```python
from build123d import *

# Parameters (mm, degrees)
SKETCH3_W           = 110
SKETCH3_H           = 180
BOSS_EXTRUDE1_DEPTH = 3
CUT_EXTRUDE1_REACH  = 107.518
SKETCH4_W           = 35
SKETCH4_H           = 55
CUT_EXTRUDE2_REACH  = 107.518
SKETCH5_R           = 1.5
FILLET1_R           = 10
FILLET2_R           = 10
SKETCH9_W           = 35
SKETCH9_H           = 3
BOSS_EXTRUDE2_DEPTH = 18.556788
BOSS_EXTRUDE3_START = -16.676438017
BOSS_EXTRUDE3_DEPTH = 35
CUT_EXTRUDE3_REACH  = 124.809
SKETCH16_W          = 10
SKETCH16_H          = 40
CHAMFER1_SIZE       = 10


# Read off the part's stored shape, not the designer's step: Boss-Extrude3
with BuildPart() as part:
    # Sketch3 → Boss-Extrude1 (new body)
    with BuildSketch(Plane(origin=(0, 0, 0), x_dir=(1, 0, 0), z_dir=(0, 1, 0))):
        Rectangle(SKETCH3_W, SKETCH3_H)
    extrude(amount=BOSS_EXTRUDE1_DEPTH)

    # Sketch4 → Cut-Extrude1 (cut, up to next)
    with BuildSketch(Plane(origin=(0, 3, 0), x_dir=(1, 0, 0), z_dir=(0, 1, 0)), mode=Mode.PRIVATE) as cut_extrude1_sk1:
        with Locations((0.823561983, -62.5)):
            Rectangle(SKETCH4_W, SKETCH4_H)
    cut_extrude1_tool1 = extrude(cut_extrude1_sk1.sketch, amount=-CUT_EXTRUDE1_REACH, mode=Mode.PRIVATE) & part.part
    add(cut_extrude1_tool1.solids().sort_by_distance((0.823562, 3, 62.5))[0], mode=Mode.SUBTRACT)

    # Sketch5 → Cut-Extrude2 (cut, up to next)
    with BuildSketch(Plane(origin=(0, 3, 0), x_dir=(1, 0, 0), z_dir=(0, 1, 0)), mode=Mode.PRIVATE) as cut_extrude2_sk1:
        with Locations(Location((37, 55, 0), (0, 0, 270))):
            Circle(SKETCH5_R)
    cut_extrude2_tool1 = extrude(cut_extrude2_sk1.sketch, amount=-CUT_EXTRUDE2_REACH, mode=Mode.PRIVATE) & part.part
    # Sketch5 → Cut-Extrude2 (cut, up to next)
    with BuildSketch(Plane(origin=(0, 3, 0), x_dir=(1, 0, 0), z_dir=(0, 1, 0)), mode=Mode.PRIVATE) as cut_extrude2_sk2:
        with Locations(Location((-37, 55, 0), (0, 0, 270))):
            Circle(SKETCH5_R)
    cut_extrude2_tool2 = extrude(cut_extrude2_sk2.sketch, amount=-CUT_EXTRUDE2_REACH, mode=Mode.PRIVATE) & part.part
    add(cut_extrude2_tool1.solids().sort_by_distance((37, 3, -55))[0], mode=Mode.SUBTRACT)
    add(cut_extrude2_tool2.solids().sort_by_distance((-37, 3, -55))[0], mode=Mode.SUBTRACT)

    # Fillet1
    fillet1_edges = [part.edges().sort_by_distance(p)[0] for p in [
        (-55, 1.5, 90),
    ]]
    fillet(fillet1_edges, radius=FILLET1_R)

    # Fillet2
    fillet2_edges = [part.edges().sort_by_distance(p)[0] for p in [
        (55, 1.5, 90),
    ]]
    fillet(fillet2_edges, radius=FILLET2_R)

    # Sketch9 → Boss-Extrude2 (add)
    with BuildSketch(Plane(origin=(0, 3, 0), x_dir=(1, 0, 0), z_dir=(0, 1, 0))):
        with Locations((0.823561983, -33.5)):
            Rectangle(SKETCH9_W, SKETCH9_H)
    extrude(amount=BOSS_EXTRUDE2_DEPTH)

    # Boss-Extrude3 outline → Boss-Extrude3 (add)
    with BuildSketch(Plane.YZ.offset(BOSS_EXTRUDE3_START)):
        with BuildLine():
            ThreePointArc((21.556787547, 32), (50.241297741, 69.962903968), (12.278393773, 98.647414162))
            Line((12.278393773, 98.647414162), (12.278393773, 95.647414162))
            ThreePointArc((12.278393773, 95.647414162), (47.241297741, 69.962903968), (21.556787547, 35))
            Line((21.556787547, 35), (21.556787547, 32))
        make_face()
    extrude(amount=BOSS_EXTRUDE3_DEPTH)

    # Sketch16 → Cut-Extrude3 (cut, up to next)
    with BuildSketch(Plane(origin=(0, 3, 0), x_dir=(1, 0, 0), z_dir=(0, 1, 0)), mode=Mode.PRIVATE) as cut_extrude3_sk1:
        with Locations((50, 55)):
            Rectangle(SKETCH16_W, SKETCH16_H)
    cut_extrude3_tool1 = extrude(cut_extrude3_sk1.sketch, amount=-CUT_EXTRUDE3_REACH, mode=Mode.PRIVATE) & part.part
    # Sketch16 → Cut-Extrude3 (cut, up to next)
    with BuildSketch(Plane(origin=(0, 3, 0), x_dir=(1, 0, 0), z_dir=(0, 1, 0)), mode=Mode.PRIVATE) as cut_extrude3_sk2:
        with Locations((-50, 55)):
            Rectangle(SKETCH16_W, SKETCH16_H)
    cut_extrude3_tool2 = extrude(cut_extrude3_sk2.sketch, amount=-CUT_EXTRUDE3_REACH, mode=Mode.PRIVATE) & part.part
    add(cut_extrude3_tool1.solids().sort_by_distance((50, 3, -55))[0], mode=Mode.SUBTRACT)
    add(cut_extrude3_tool2.solids().sort_by_distance((-50, 3, -55))[0], mode=Mode.SUBTRACT)

    # Chamfer1
    chamfer1_edges = [part.edges().sort_by_distance(p)[0] for p in [
        (-55, 1.5, -90),
        (55, 1.5, -90),
    ]]
    chamfer(chamfer1_edges, length=CHAMFER1_SIZE)


solid = part.part
```
Could you check a few things on this model? Use its own coordinates, in mm. A direction names the side the tool comes from. Give positions to 0.01 mm unless a question says otherwise; leave off trailing zeros. Order: outer loops, then holes, each group sorted by start corner. A loop starts at its lowest first (then second) coordinate and runs counter-clockwise, first axis right, second up.
Q1. If I drill on line 1 along X through (y, z) = (2.35, -55); line 2 along Y through (x, z) = (-18, 51); line 3 along Z through (x, y) = (-10, 4.5), over which ranges is the centre line in solid material (lowest first)?
Q2. For faces 1 (the flat face through (18.324, 48, 63)), 2 (the flat face through (-16.676, 48, 63)), 3 (the flat face through (1, 12, 32)), which set-ups out of +Z, -Z, +X, -X, +Y, -Y let a thin tool reach every point of the face, with its end or its side?
Q3. Suppose I cut it at D-D, the plane y = 40. Write out the boundary of the cut face in (x, z), and give its area (3 significant figures).
Q4. We'd pull the mould along Z, two halves only. Please class faces 4 (the cylindrical face through (0.58, 47.13, 70.63)), 5 (the flat face through (-50, 1, -85)), 6 (the flat face through (-1, 0, -1)): +Z half, -Z half, draft (parallel to the pull), parting line (faces both ways), or undercut.
Q5. Suppose I cut it at A-A, the plane y = 24. Write out the boundary of the cut face in (x, z), and give its area (3 significant figures).
Q6. I'm going to push flat-ended pins straight in: P1, Ø2.5, axis at x = -51, y = 1.5, coming from the -Z side; P2, Ø17, axis at x = -0.5, y = 9.5, coming from the +Z side; P3, Ø1.5, axis at y = 12.5, z = 31.5, coming from the +X side. Where does each tip first touch, or does it pass through?
Q7. Suppose I cut it at B-B, the plane z = 69.5. Write out the boundary of the cut face in (x, y), and give its area (3 significant figures).
Solution:
1. line 1: x = -45 to -38.5, -35.5 to 35.5, 38.5 to 45
1. line 2: y = 0 to 3
1. line 3: z = 32 to 35
2. face 1: +Z, -Z, +X, +Y
2. face 2: +Z, -Z, -X, +Y
2. face 3: -Z, +X, -X, +Y
3. outline: (-16.68, 40.85) - (18.32, 40.85) - (18.32, 45.12) - (-16.68, 45.12) - close; (-16.68, 85.53) - (18.32, 85.53) - (18.32, 89.8) - (-16.68, 89.8) - close
3. area: 299 mm2
4. face 4: undercut
4. face 5: -Z half
4. face 6: draft
5. outline: (-16.68, 32.43) - (18.32, 32.43) - (18.32, 35.48) - (-16.68, 35.48) - close; (-16.68, 95.17) - (18.32, 95.17) - (18.32, 98.21) - (-16.68, 98.21) - close
5. area: 213 mm2
6. P1: stops at z = -85.25
6. P2: stops at z = 98.97
6. P3: stops at x = 18.32
7. outline: (-55, 0) - (-16.68, 0) - (-16.68, 3) - (-55, 3) - close; (-16.68, 47.31) - (18.32, 47.31) - (18.32, 50.3) - (-16.68, 50.3) - close; (18.32, 0) - (55, 0) - (55, 3) - (18.32, 3) - close
7. area: 330 mm2
